Geometry check sheet. Reference: the model listing, model coordinates, mm. Round coordinates to 2 decimals unless told otherwise and drop trailing zeros.
(1) Material ranges on line 1 along X through (y, z) = (75, -3.75); line 2 along X through (y, z) = (6, 10.75); line 3 along Y through (x, z) = (47.5, 8), recorded low to high.
(2) Release check for a two-part mould opening along Z. For faces 1 (the face through (32.4, 80.8, 12.8)), 2 (the face through (32, 1, 1)) record: +Z half, -Z half, draft (parallel to the pull), parting line (faces both ways), or undercut.
(3) Go/stop test with flat-tipped pins: pin 1 (1.5 mm diameter, centred on y = 48, z = -7.5, fed in from -X); pin 2 (3 mm diameter, centred on x = 47.5, y = 19, fed in from -Z); pin 3 (5 mm diameter, centred on x = 46, z = 5, fed in from -Y); pin 4 (2 mm diameter, centred on y = 36.5, z = -6, fed in from +X). Record where each tip stops, or that it passes through.
from build123d import *


with BuildPart() as part:
    # Bottom → Magazine Body section 0
    with BuildSketch(Plane(origin=(0, 0, 0), x_dir=(1, 0, 0), z_dir=(0, 1, 0))):
        with BuildLine():
            Line((-7.648338397, 10.646601169), (-7.648338397, -14.253398831))
            Line((-7.648338397, -14.253398831), (73.151661603, -12.299887169))
            Line((73.151661603, -12.299887169), (73.151661603, 8.700112831))
            Line((73.151661603, 8.700112831), (-7.648338397, 10.646601169))
        make_face()
    # Top → Magazine Body section 1
    with BuildSketch(Plane(origin=(0, 80.8, 0), x_dir=(1, 0, 0), z_dir=(0, 1, 0))):
        with BuildLine():
            Line((73.001661603, -12.153469905), (73.001661603, 8.553682842))
            Line((73.001661603, 8.553682842), (-7.498338397, 10.49294412))
            Line((-7.498338397, 10.49294412), (-7.498338397, -14.099728429))
            Line((-7.498338397, -14.099728429), (73.001661603, -12.153469905))
        make_face()
    loft()

    # Sketch4 → Magazine Inner Cut section 0
    with BuildSketch(Plane(origin=(0, 1, 0), x_dir=(-1, 0, 0), z_dir=(0, -1, 0))):
        with BuildLine():
            Line((6.648338397, -13.228929483), (6.648338397, 9.62222084))
            Line((6.648338397, 9.62222084), (-72.151661603, 7.723912906))
            Line((-72.151661603, 7.723912906), (-72.151661603, -11.32377207))
            Line((-72.151661603, -11.32377207), (6.648338397, -13.228929483))
        make_face()
    # Sketch5 → Magazine Inner Cut section 1
    with BuildSketch(Plane(origin=(0, 80.8, 0), x_dir=(1, 0, 0), z_dir=(0, 1, 0))):
        with BuildLine():
            Line((72.001661603, -11.177354805), (72.001661603, 7.577482917))
            Line((72.001661603, 7.577482917), (-6.498338397, 9.468563791))
            Line((-6.498338397, 9.468563791), (-6.498338397, -13.07525908))
            Line((-6.498338397, -13.07525908), (72.001661603, -11.177354805))
        make_face()
    loft(mode=Mode.SUBTRACT)


solid = part.part
Answer below:
1. line 1: x = -7.51 to -6.51, 72.01 to 73.01
1. line 2: x = -7.64 to -6.64, 72.14 to 73.14
1. line 3: y = 0 to 1
2. face 1: draft
2. face 2: undercut
3. pin 1: stops at x = -7.56
3. pin 2: stops at z = -9.32
3. pin 3: stops at y = 0
3. pin 4: stops at x = 73.09
